```python
from build123d import *

# Parameters (mm, degrees)
SKETCH1_W                     = 63
SKETCH1_H                     = 63
BOSS_EXTRUDE2_DEPTH           = 25
SKETCH1_4_W                   = 59
SKETCH1_4_H                   = 55
CUT_EXTRUDE1_DEPTH            = 23
SKETCH4_W                     = 2
SKETCH4_H                     = 55
BOSS_EXTRUDE3_DEPTH           = 10
FILLET1_R                     = 2
SKETCH5_W                     = 2
SKETCH5_H                     = 63
CUT_EXTRUDE3_DEPTH            = 93.536479293
SKETCH6_W                     = 2.2
SKETCH6_H                     = 2.2
CUT_EXTRUDE4_DEPTH            = 59
SKETCH7_W                     = 10
SKETCH7_H                     = 10
CUT_EXTRUDE5_DEPTH            = 2.5
CUT_EXTRUDE6_DEPTH            = 11.5
CUT_EXTRUDE6_DEPTH_BACK       = 1.5
SKETCH8_R                     = 0.875
SKETCH9_W                     = 10
SKETCH9_H                     = 10
CUT_EXTRUDE7_DEPTH            = 2.5
CUT_EXTRUDE8_DEPTH            = 11.5
CUT_EXTRUDE8_DEPTH_BACK       = 1.5
SKETCH10_R                    = 0.875
CUT_EXTRUDE9_DEPTH            = 2
CUT_EXTRUDE10_DEPTH           = 2
FILLET2_R                     = 0.3
CUT_EXTRUDE12_REACH           = 94.536
CUT_EXTRUDE13_REACH           = 77.606
SKETCH15_W                    = 5
SKETCH15_H                    = 10
FILLET3_R                     = 1
SKETCH18_R                    = 2.4
CUT_EXTRUDE16_DEPTH           = 10
CUT_EXTRUDE16_DRAFT           = 2
SKETCH18_R_2                  = 5.5
CUT_EXTRUDE16_PROFILE_2_DEPTH = 10
CUT_EXTRUDE16_PROFILE_2_DRAFT = 2
SKETCH18_R_3                  = 1
CUT_EXTRUDE16_PROFILE_3_DEPTH = 10
CUT_EXTRUDE16_PROFILE_3_DRAFT = 2
CUT_EXTRUDE16_PROFILE_4_DEPTH = 10
CUT_EXTRUDE16_PROFILE_4_DRAFT = 2
SKETCH19_R                    = 2.469841539
BOSS_EXTRUDE4_DEPTH           = 6
SKETCH13_R                    = 0.6
CUT_EXTRUDE17_DEPTH           = 6


with BuildPart() as part:
    # Sketch1 → Boss-Extrude2 (new body)
    with BuildSketch(Plane(origin=(0, 0, 0), x_dir=(1, 0, 0), z_dir=(0, 1, 0))):
        with Locations((31.5, 31.5)):
            Rectangle(SKETCH1_W, SKETCH1_H)
    extrude(amount=BOSS_EXTRUDE2_DEPTH)

    # Sketch1<4> → Cut-Extrude1 (cut)
    with BuildSketch(Plane(origin=(0, 0, 0), x_dir=(1, 0, 0), z_dir=(0, 1, 0))):
        with Locations((31.5, 31.5)):
            Rectangle(SKETCH1_4_W, SKETCH1_4_H)
    extrude(amount=CUT_EXTRUDE1_DEPTH, mode=Mode.SUBTRACT)

    # Sketch4 → Boss-Extrude3 (add)
    with BuildSketch(Plane.XZ.offset(-23)):
        with Locations((30.5, -31.5)):
            Rectangle(SKETCH4_W, SKETCH4_H)
    extrude(amount=BOSS_EXTRUDE3_DEPTH)

    # Fillet1
    fillet1_edges = [part.edges().sort_by_distance(p)[0] for p in [
        (63, 25, -31.5),
        (31.5, 25, 0),
        (0, 25, -31.5),
        (0, 12.5, 0),
        (63, 12.5, 0),
        (63, 12.5, -63),
        (0, 12.5, -63),
        (31.5, 25, -63),
    ]]
    fillet(fillet1_edges, radius=FILLET1_R)

    # Sketch5 → Cut-Extrude3 (cut, through all)
    with BuildSketch(Plane(origin=(0, 0, 0), x_dir=(-1, 0, 0), z_dir=(0, -1, 0))):
        with Locations((-1, 31.5)):
            Rectangle(SKETCH5_W, SKETCH5_H)
    extrude(amount=-CUT_EXTRUDE3_DEPTH, mode=Mode.SUBTRACT)

    # Sketch6 → Cut-Extrude4 (cut)
    with BuildSketch(Plane.ZY.offset(-2)):
        with Locations((-2.9, 1.85)):
            Rectangle(SKETCH6_W, SKETCH6_H)
        with Locations((-60.1, 1.85)):
            Rectangle(SKETCH6_W, SKETCH6_H)
    extrude(amount=-CUT_EXTRUDE4_DEPTH, mode=Mode.SUBTRACT)

    # Sketch7 → Cut-Extrude5 (cut)
    with BuildSketch(Plane(origin=(0, 0, -63), x_dir=(-1, 0, 0), z_dir=(0, 0, -1))):
        with Locations((-7, 12)):
            Rectangle(SKETCH7_W, SKETCH7_H)
    extrude(amount=-CUT_EXTRUDE5_DEPTH, mode=Mode.SUBTRACT)

    # Sketch8 → Cut-Extrude6 (cut, two sides: drawn at the far end of the back side and taken through both)
    with BuildSketch(Plane(origin=(0, 7, 0), x_dir=(1, 0, 0), z_dir=(0, 1, 0)).offset(-CUT_EXTRUDE6_DEPTH_BACK)):
        with Locations(Location((10, 61.5, 0), (0, 0, 270))):
            Circle(SKETCH8_R)
    extrude(amount=CUT_EXTRUDE6_DEPTH + CUT_EXTRUDE6_DEPTH_BACK, mode=Mode.SUBTRACT)

    # Sketch9 → Cut-Extrude7 (cut)
    with BuildSketch(Plane.XY):
        with Locations((7, 12)):
            Rectangle(SKETCH9_W, SKETCH9_H)
    extrude(amount=-CUT_EXTRUDE7_DEPTH, mode=Mode.SUBTRACT)

    # Sketch10 → Cut-Extrude8 (cut, two sides: drawn at the far end of the back side and taken through both)
    with BuildSketch(Plane(origin=(0, 7, 0), x_dir=(1, 0, 0), z_dir=(0, 1, 0)).offset(-CUT_EXTRUDE8_DEPTH_BACK)):
        with Locations((10, 1.5)):
            Circle(SKETCH10_R)
    extrude(amount=CUT_EXTRUDE8_DEPTH + CUT_EXTRUDE8_DEPTH_BACK, mode=Mode.SUBTRACT)

    # Sketch11 → Cut-Extrude9 (cut)
    with BuildSketch(Plane(origin=(0, 0, -63), x_dir=(-1, 0, 0), z_dir=(0, 0, -1))):
        with BuildLine():
            Line((-9.122986176, 7), (-10.8, 7))
            add(Edge.make_bspline(
                [(-10.8, 7), (-9.980201359, 6.395551325), (-9.122986176, 7)],
                knots=[0, 0, 0, 1, 1, 1], degree=2))
        make_face()
        with BuildLine():
            Line((-9.122986176, 17), (-10.8, 17))
            add(Edge.make_bspline(
                [(-10.8, 17), (-9.980201359, 17.604448675), (-9.122986176, 17)],
                knots=[0, 0, 0, 1, 1, 1], degree=2))
        make_face()
    extrude(amount=-CUT_EXTRUDE9_DEPTH, mode=Mode.SUBTRACT)

    # Sketch12 → Cut-Extrude10 (cut)
    with BuildSketch(Plane.XY):
        with BuildLine():
            Line((11, 7), (9.120131213, 7))
            add(Edge.make_bspline(
                [(11, 7), (10.05659536, 6.399803182), (9.120131213, 7)],
                knots=[0, 0, 0, 1, 1, 1], degree=2))
        make_face()
        with BuildLine():
            Line((11, 17), (9.120131213, 17))
            add(Edge.make_bspline(
                [(11, 17), (10.05659536, 17.600196818), (9.120131213, 17)],
                knots=[0, 0, 0, 1, 1, 1], degree=2))
        make_face()
    extrude(amount=-CUT_EXTRUDE10_DEPTH, mode=Mode.SUBTRACT)

    # Fillet2
    fillet2_edges = [part.edges().sort_by_distance(p)[0] for p in [
        (31.5, 2.95, -59),
        (2, 0.75, -60.1),
        (2, 1.85, -61.2),
        (31.5, 0.75, -61.2),
        (31.5, 2.95, -61.2),
        (2, 2.95, -60.1),
        (2, 2.95, -2.9),
        (31.5, 2.95, -4),
        (31.5, 2.95, -1.8),
        (31.5, 0.75, -1.8),
        (2, 0.75, -2.9),
        (2, 1.85, -1.8),
    ]]
    fillet(fillet2_edges, radius=FILLET2_R)

    # Sketch14 → Cut-Extrude12 (cut, up to next)
    with BuildSketch(Plane(origin=(0, 0, -63), x_dir=(-1, 0, 0), z_dir=(0, 0, -1)), mode=Mode.PRIVATE) as cut_extrude12_sk1:
        with BuildLine():
            Line((-39, 14.7), (-45, 14.7))
            ThreePointArc((-45, 14.7), (-48.25, 17.95), (-45, 21.2))
            Line((-45, 21.2), (-39, 21.2))
            ThreePointArc((-39, 21.2), (-35.75, 17.95), (-39, 14.7))
        make_face()
    cut_extrude12_tool1 = extrude(cut_extrude12_sk1.sketch, amount=-CUT_EXTRUDE12_REACH, mode=Mode.PRIVATE) & part.part
    add(cut_extrude12_tool1.solids().sort_by_distance((42, 17.95, -63))[0], mode=Mode.SUBTRACT)

    # Sketch15 → Cut-Extrude13 (cut, up to next)
    with BuildSketch(Plane.ZY.offset(-29.5), mode=Mode.PRIVATE) as cut_extrude13_sk1:
        with Locations((-6.5, 18)):
            Rectangle(SKETCH15_W, SKETCH15_H)
    cut_extrude13_tool1 = extrude(cut_extrude13_sk1.sketch, amount=-CUT_EXTRUDE13_REACH, mode=Mode.PRIVATE) & part.part
    add(cut_extrude13_tool1.solids().sort_by_distance((29.5, 18, -6.5))[0], mode=Mode.SUBTRACT)

    # Fillet3
    fillet3_edges = [part.edges().sort_by_distance(p)[0] for p in [
        (29.5, 13, -34),
        (30.5, 13, -9),
        (29.5, 18, -59),
        (31.5, 18, -59),
        (30.5, 13, -59),
        (31.5, 13, -34),
    ]]
    fillet(fillet3_edges, radius=FILLET3_R - 0.0001)  # a hair under: the kernel refuses the full size


with BuildPart() as cut_extrude16_tool:
    # Sketch18 → Cut-Extrude16 (with draft: the straight prism first)
    with BuildSketch(Plane(origin=(63, 0, 0), x_dir=(0, 0, -1), z_dir=(1, 0, 0))):
        with Locations((55.2, 8)):
            Circle(SKETCH18_R)
    extrude(amount=-CUT_EXTRUDE16_DEPTH)
    # Cut-Extrude16: the draft: its side faces are tilted about the plane it starts from
    cut_extrude16_sides = [cut_extrude16_tool.faces().sort_by_distance(p)[0] for p in [
        (58, 8, -52.8),
    ]]
    draft(cut_extrude16_sides, Plane(origin=(63, 0, 0), x_dir=(0, 0, -1), z_dir=(1, 0, 0)), CUT_EXTRUDE16_DRAFT)


with BuildPart() as part_1:
    add(part.part)

    # Cut-Extrude16: cut by cut_extrude16_tool
    add(cut_extrude16_tool.part, mode=Mode.SUBTRACT)


with BuildPart() as cut_extrude16_profile_2_tool:
    # Sketch18 → Cut-Extrude16 profile 2 (with draft: the straight prism first)
    with BuildSketch(Plane(origin=(63, 0, 0), x_dir=(0, 0, -1), z_dir=(1, 0, 0))):
        with Locations((42, 11.5)):
            Circle(SKETCH18_R_2)
    extrude(amount=-CUT_EXTRUDE16_PROFILE_2_DEPTH)
    # Cut-Extrude16 profile 2: the draft: its side faces are tilted about the plane it starts from
    cut_extrude16_profile_2_sides = [cut_extrude16_profile_2_tool.faces().sort_by_distance(p)[0] for p in [
        (58, 11.5, -36.5),
    ]]
    draft(cut_extrude16_profile_2_sides, Plane(origin=(63, 0, 0), x_dir=(0, 0, -1), z_dir=(1, 0, 0)), CUT_EXTRUDE16_PROFILE_2_DRAFT)


with BuildPart() as part_2:
    add(part_1.part)

    # Cut-Extrude16 profile 2: cut by cut_extrude16_profile_2_tool
    add(cut_extrude16_profile_2_tool.part, mode=Mode.SUBTRACT)


with BuildPart() as cut_extrude16_profile_3_tool:
    # Sketch18 → Cut-Extrude16 profile 3 (with draft: the straight prism first)
    with BuildSketch(Plane(origin=(63, 0, 0), x_dir=(0, 0, -1), z_dir=(1, 0, 0))):
        with Locations((44.75, 2.5)):
            Circle(SKETCH18_R_3)
    extrude(amount=-CUT_EXTRUDE16_PROFILE_3_DEPTH)
    # Cut-Extrude16 profile 3: the draft: its side faces are tilted about the plane it starts from
    cut_extrude16_profile_3_sides = [cut_extrude16_profile_3_tool.faces().sort_by_distance(p)[0] for p in [
        (58, 2.5, -43.75),
    ]]
    draft(cut_extrude16_profile_3_sides, Plane(origin=(63, 0, 0), x_dir=(0, 0, -1), z_dir=(1, 0, 0)), CUT_EXTRUDE16_PROFILE_3_DRAFT)


with BuildPart() as part_3:
    add(part_2.part)

    # Cut-Extrude16 profile 3: cut by cut_extrude16_profile_3_tool
    add(cut_extrude16_profile_3_tool.part, mode=Mode.SUBTRACT)


with BuildPart() as cut_extrude16_profile_4_tool:
    # Sketch18 → Cut-Extrude16 profile 4 (with draft: the straight prism first)
    with BuildSketch(Plane(origin=(63, 0, 0), x_dir=(0, 0, -1), z_dir=(1, 0, 0))):
        with Locations((6.5, 2.5)):
            Circle(SKETCH18_R_3)
    extrude(amount=-CUT_EXTRUDE16_PROFILE_4_DEPTH)
    # Cut-Extrude16 profile 4: the draft: its side faces are tilted about the plane it starts from
    cut_extrude16_profile_4_sides = [cut_extrude16_profile_4_tool.faces().sort_by_distance(p)[0] for p in [
        (58, 2.5, -5.5),
    ]]
    draft(cut_extrude16_profile_4_sides, Plane(origin=(63, 0, 0), x_dir=(0, 0, -1), z_dir=(1, 0, 0)), CUT_EXTRUDE16_PROFILE_4_DRAFT)


with BuildPart() as part_4:
    add(part_3.part)

    # Cut-Extrude16 profile 4: cut by cut_extrude16_profile_4_tool
    add(cut_extrude16_profile_4_tool.part, mode=Mode.SUBTRACT)

    # Sketch19 → Boss-Extrude4 (add)
    with BuildSketch(Plane.ZY.offset(-61)):
        with BuildLine():
            ThreePointArc((-59, 6.7510004), (-54.567544468, 4.050316468), (-51.2, 8))
            ThreePointArc((-51.2, 8), (-54.567544468, 11.949683532), (-59, 9.2489996))
            Line((-59, 9.2489996), (-59, 6.7510004))
        make_face()
        with Locations((-55.2, 8)):
            Circle(SKETCH19_R, mode=Mode.SUBTRACT)
    extrude(amount=BOSS_EXTRUDE4_DEPTH)

    # Sketch13 → Cut-Extrude17 (cut)
    with BuildSketch(Plane(origin=(0, 23, 0), x_dir=(-1, 0, 0), z_dir=(0, -1, 0))):
        with Locations(Location((-34.5, 57, 0), (0, 0, 90))):
            Circle(SKETCH13_R)
        with Locations(Location((-49.5, 57, 0), (0, 0, 90))):
            Circle(SKETCH13_R)
        with Locations(Location((-49.5, 16.5, 0), (0, 0, 90))):
            Circle(SKETCH13_R)
        with Locations(Location((-34.5, 16.5, 0), (0, 0, 90))):
            Circle(SKETCH13_R)
    extrude(amount=-CUT_EXTRUDE17_DEPTH, mode=Mode.SUBTRACT)


solid = part_4.part
```
The listing builds one solid part. Answer for the finished solid, in the listing's coordinates (mm). A direction names the side the tool comes from. Round coordinates to 2 decimals unless told otherwise and drop trailing zeros. Write each loop counter-clockwise with the first axis right and the second up, starting at its lowest first coordinate (ties: lowest second). Pieces come first, ordered by that corner, then holes. Notation, with made-up numbers: (27.5, 85) -> (36.5, 85) arc R9 cw to (36.5, 89) -> close; hole circle Ø10 at (59.5, 23). An arc over 180 degrees is marked (long way). Answer as a JSON object with one key per item and string values. Group by question number.
Q1. Determine the mould class of faces 1 (the face through (31, 13, -4)), 2 (the face through (48.25, 17.88, -61.03)), 3 (the face through (31.91, 24.4, -0.57)) for opening direction Y: pulls with the +Y half, pulls with the -Y half, needs draft (parallel to the pull), parting line crosses it, or undercut.
Q2. Straight lines are drawn through the part: line 1 along Z through (x, y) = (10, 6) (3 decimals); line 2 along X through (y, z) = (14.5, -55); line 3 along X through (y, z) = (17.75, -61.5) (1 decimal). For each, find the intervals that lie inside material, in ascending order.
Q3. Section D-D (z = -45) is taken. Count the separate pieces of the cut face and the enclosed holes in it, plus the area to 3 significant figures.
Q4. Each of these flat-tipped pins is pushed along its axis until it touches: pin 1 Ø5 at (y, z) = (5.5, -49) entering from -X; pin 2 Ø12 at (x, z) = (52, -37.5) entering from -Y; pin 3 Ø1.1 at (x, z) = (34.5, -16.5) entering from -Y; pin 4 Ø4 at (y, z) = (15, -12.5) entering from -X. Where does it stop, or does it pass through?
Q5. Section B-B (x = 56) is taken. Write down the section's boundary in (y, z), plus the area to 3 significant figures.
Q6. Section A-A (x = 18) is taken. Write down the section's boundary in (y, z).
Q7. Which of the six approach directions +Z, -Z, +X, -X, +Y, -Y give full straight-line access (tool end or side, diameter ignored) to faces 4 (the face through (31, 0.75, -3)), 5 (the face through (35.75, 18.02, -61.03)), 6 (the face through (10, 5.5, -2)), 7 (the face through (6, 7, -1))?
Check values:
{
 "1": {"face 1": "needs draft", "face 2": "undercut", "face 3": "pulls with the +Y half"},
 "2": {"line 1": "-63 to -62.375, -60.625 to -59, -4 to -2.375, -0.625 to 0", "line 2": "29.5 to 31.5, 61 to 63", "line 3": "2 to 9.1, 10.9 to 35.8, 48.2 to 62.9"},
 "3": {"separate pieces": "3", "enclosed holes": "0", "area": "164 mm^2"},
 "4": {"pin 1": "x = 61", "pin 2": "y = 23", "pin 3": "through", "pin 4": "x = 29.5"},
 "5": {"outline": "(0, -63) -> (23, -63) arc R2 ccw to (25, -61) -> (25, -2) arc R2 ccw to (23, 0) -> (0, 0) -> (0, -4) -> (0.75, -4) -> (0.75, -2.1) arc R0.3 cw to (1.05, -1.8) -> (2.65, -1.8) arc R0.3 cw to (2.95, -2.1) -> (2.95, -3.7) arc R0.3 ccw to (3.25, -4) -> (23, -4) -> (23, -59) -> (9.25, -59) arc R4 ccw (long way) to (6.75, -59) -> (3.25, -59) arc R0.3 ccw to (2.95, -59.3) -> (2.95, -60.9) arc R0.3 cw to (2.65, -61.2) -> (1.05, -61.2) arc R0.3 cw to (0.75, -60.9) -> (0.75, -59) -> (0, -59) -> close; hole circle Ø4.94 at (8, -55.2)", "area": "329 mm^2"},
 "6": {"outline": "(0, -63) -> (23, -63) arc R2 ccw to (25, -61) -> (25, -2) arc R2 ccw to (23, 0) -> (0, 0) -> (0, -4) -> (0.75, -4) -> (0.75, -2.1) arc R0.3 cw to (1.05, -1.8) -> (2.65, -1.8) arc R0.3 cw to (2.95, -2.1) -> (2.95, -3.7) arc R0.3 ccw to (3.25, -4) -> (23, -4) -> (23, -59) -> (3.25, -59) arc R0.3 ccw to (2.95, -59.3) -> (2.95, -60.9) arc R0.3 cw to (2.65, -61.2) -> (1.05, -61.2) arc R0.3 cw to (0.75, -60.9) -> (0.75, -59) -> (0, -59) -> close"},
 "7": {"face 4": "-X", "face 5": "-Z", "face 6": "none", "face 7": "+Z, -X"}
}
